Geometry: see drawing. Coordinates: mm, zero at the bounding-box minimum. A direction names the side the tool comes from. Coordinates: 2 decimals unless noted, no trailing zeros. Order: outer loops, then holes, each group sorted by start corner. A loop starts at its lowest first (then second) coordinate and runs counter-clockwise, first axis right, second up. Notation, with made-up numbers: (68, 68.25) -> (126, 68.25) arc R32 cw to (126, 94.25) -> close; hole circle Ø7 at (13.25, -25.75). An arc over 180 degrees is marked (long way). Use CSV: the item, a comma, the result in double quotes. Start each with the question number.
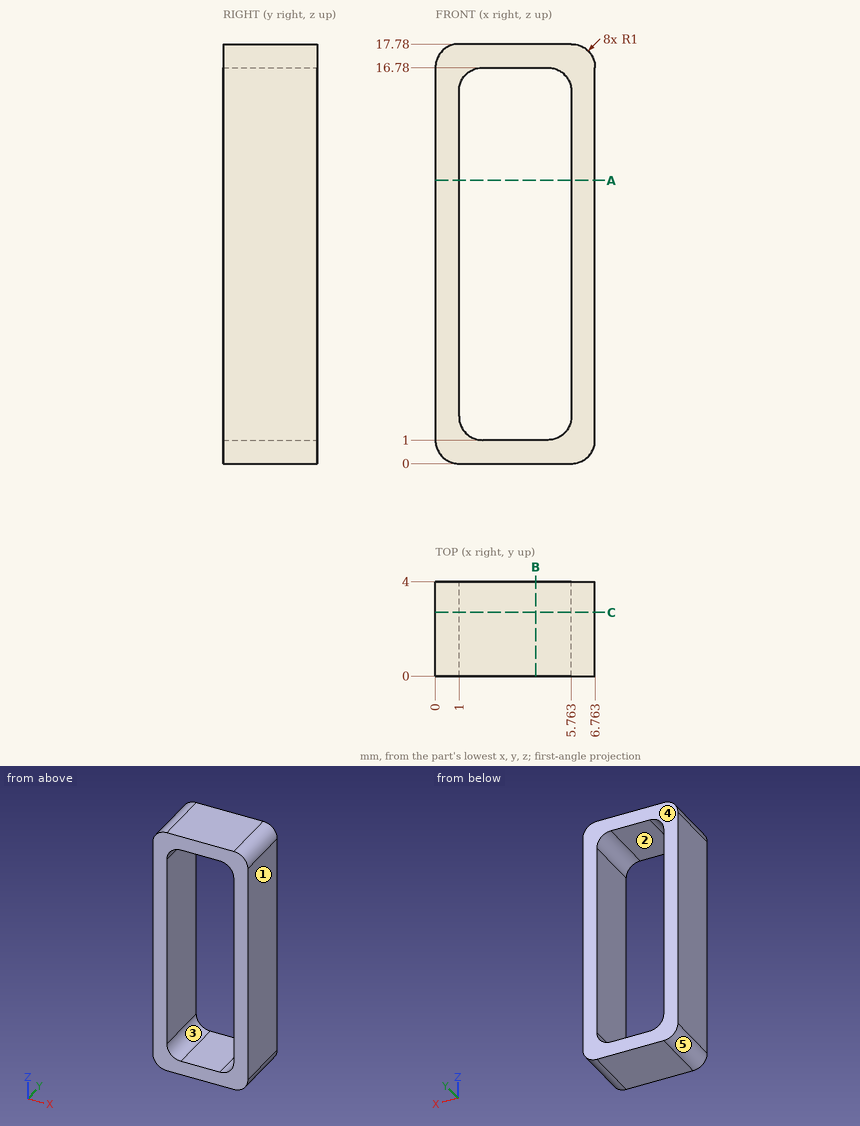
(1) Section B-B (x = 4.25). Return loops of the section in (y, z).
(2) First-contact query: pin 1 (3 mm diameter, centred on x = 3.5, z = 15.5, fed in from +Y). Flat tip, straight axial feed; report the tip coordinate or a pass-through.
(3) Mould query, pull axis Z, two halves, no side actions, for the marked faces 3, 4 and 5. Classes: pulls with the +Z half, pulls with the -Z half, needs draft (parallel to the pull), parting line crosses it, or undercut.
(4) Section A-A (z = 12). Return loops of the section in (x, y).
(5) Section C-C (y = 2.7). Return loops of the section in (x, z).
(6) Line query: line 1 (X direction, y = 0.9, z = 2.75); line 2 (Z direction, x = 4.5, y = 1.35); line 3 (X direction, y = 3.5, z = 1.75). Output: solid intervals per line, ascending. Write a range as from..to.
(7) Access query for the marked faces 1 and 2. Directions: +Z, -Z, +X, -X, +Y, -Y. A direction counts if a zero-diameter tool reaches every point of the face in a straight line with its end or side. Return the directions, or none.
Check sheet entries:
1,outline,"(0, 0) -> (4, 0) -> (4, 1) -> (0, 1) -> close; (0, 16.78) -> (4, 16.78) -> (4, 17.78) -> (0, 17.78) -> close"
2,pin 1,"stops at y = 4"
3,face 3,"undercut"
3,face 4,"needs draft"
3,face 5,"pulls with the -Z half"
4,outline,"(0, 0) -> (1, 0) -> (1, 4) -> (0, 4) -> close; (5.76, 0) -> (6.76, 0) -> (6.76, 4) -> (5.76, 4) -> close"
5,outline,"(0, 1) arc R1 ccw to (1, 0) -> (5.76, 0) arc R1 ccw to (6.76, 1) -> (6.76, 16.78) arc R1 ccw to (5.76, 17.78) -> (1, 17.78) arc R1 ccw to (0, 16.78) -> close; hole (1, 2) arc R1 ccw to (2, 1) -> (4.76, 1) arc R1 ccw to (5.76, 2) -> (5.76, 15.78) arc R1 ccw to (4.76, 16.78) -> (2, 16.78) arc R1 ccw to (1, 15.78) -> close"
6,line 1,"x = 0..1, 5.76..6.76"
6,line 2,"z = 0..1, 16.78..17.78"
6,line 3,"x = 0..1.03, 5.73..6.76"
7,face 1,"+Z, -Z, +X, +Y, -Y"
7,face 2,"+Y, -Y"
